Part print with two shaded views. Sizes in mm from the minimum x, y, z corner. Round coordinates to 2 decimals unless told otherwise and drop trailing zeros. Order: outer loops, then holes, each group sorted by start corner. A loop starts at its lowest first (then second) coordinate and runs counter-clockwise, first axis right, second up. Notation, with made-up numbers: (81, 67) -> (119, 67) arc R37 ccw to (119, 103) -> close; hole circle Ø7 at (64.5, 42.5). An arc over 180 degrees is marked (long way). Use a Markdown table: item, result. Add a question column.
Item 1: Probe L1, parallel to Y at x = 83, z = 63; L2, parallel to Z at x = 119, y = 113; L3, parallel to Y at x = 28.5, z = 68.5. List the from-to ranges inside material, lowest first.
Item 2: Slice it at A-A, the plane y = 127. Give the cut face in (x, z), plus the area to 3 significant figures.
Item 3: Slice it at B-B, the plane x = 84.5. Give the cut face in (y, z).
Item 4: Pin check, flat tip, straight feed: pin 1 (3 mm diameter, centred on x = 42, z = 106, fed in from +Y). Stop position of the tip, or through.
Item 5: Slice it at C-C, the plane z = 63.5. Give the cut face in (x, y).
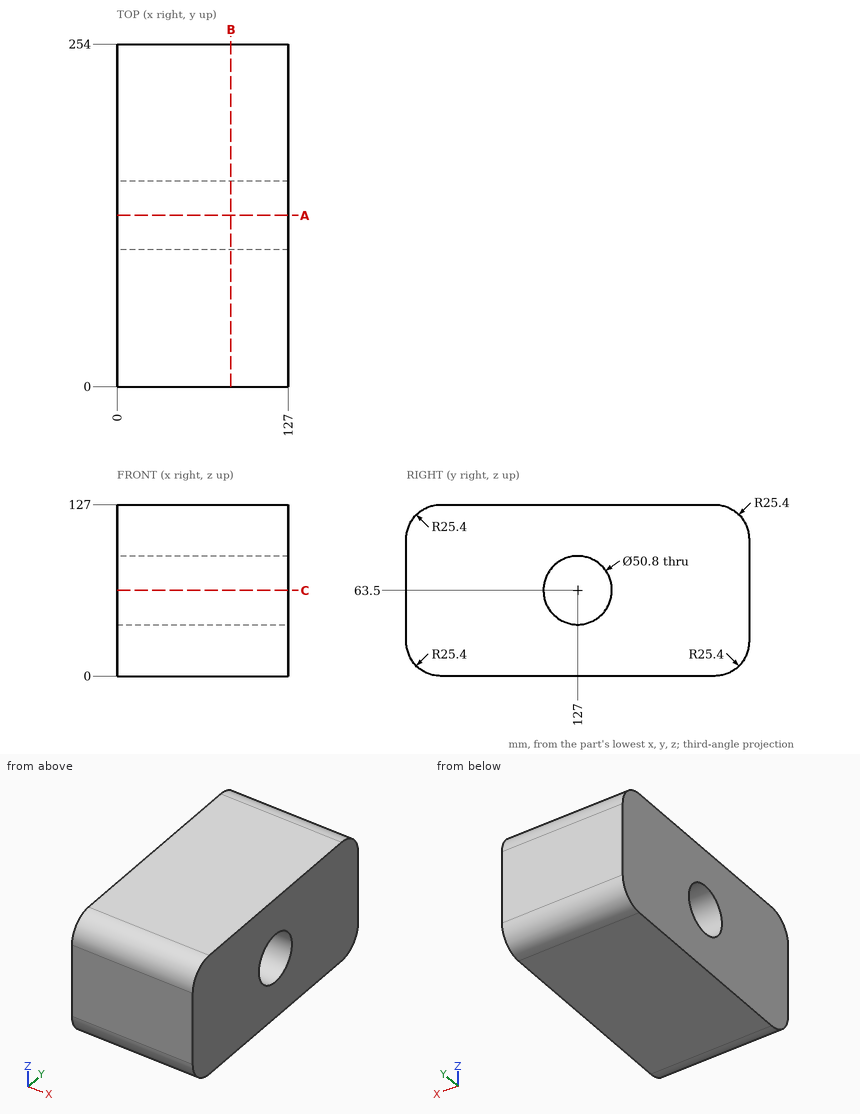
Check sheet entries:
| question | item | result |
|---|---|---|
| 1 | L1 | 0 to 101.6, 152.4 to 254 |
| 1 | L2 | 0 to 42.31, 84.69 to 127 |
| 1 | L3 | 0 to 102.1, 151.9 to 254 |
| 2 | outline | (0, 0) -> (127, 0) -> (127, 38.1) -> (0, 38.1) -> close; (0, 88.9) -> (127, 88.9) -> (127, 127) -> (0, 127) -> close |
| 2 | area | 9,680 mm2 |
| 3 | outline | (0, 25.4) arc R25.4 ccw to (25.4, 0) -> (228.6, 0) arc R25.4 ccw to (254, 25.4) -> (254, 101.6) arc R25.4 ccw to (228.6, 127) -> (25.4, 127) arc R25.4 ccw to (0, 101.6) -> close; hole circle Ø50.8 at (127, 63.5) |
| 4 | pin 1 | y = 253.83 |
| 5 | outline | (0, 0) -> (127, 0) -> (127, 101.6) -> (0, 101.6) -> close; (0, 152.4) -> (127, 152.4) -> (127, 254) -> (0, 254) -> close |
